Geometry: see drawing. Coordinates: mm, zero at the bounding-box minimum. Coordinates: 2 decimals unless noted, no trailing zeros. Order: outer loops, then holes, each group sorted by start corner. A loop starts at its lowest first (then second) coordinate and runs counter-clockwise, first axis right, second up. Notation, with made-up numbers: (-30.75, 47) -> (-16.75, 47) arc R17 ccw to (-16.75, 62) -> close; hole circle Ø2 at (33, -26.5). An arc over 180 degrees is marked (long way). Write each question's results on one line, items separated by ' | '.
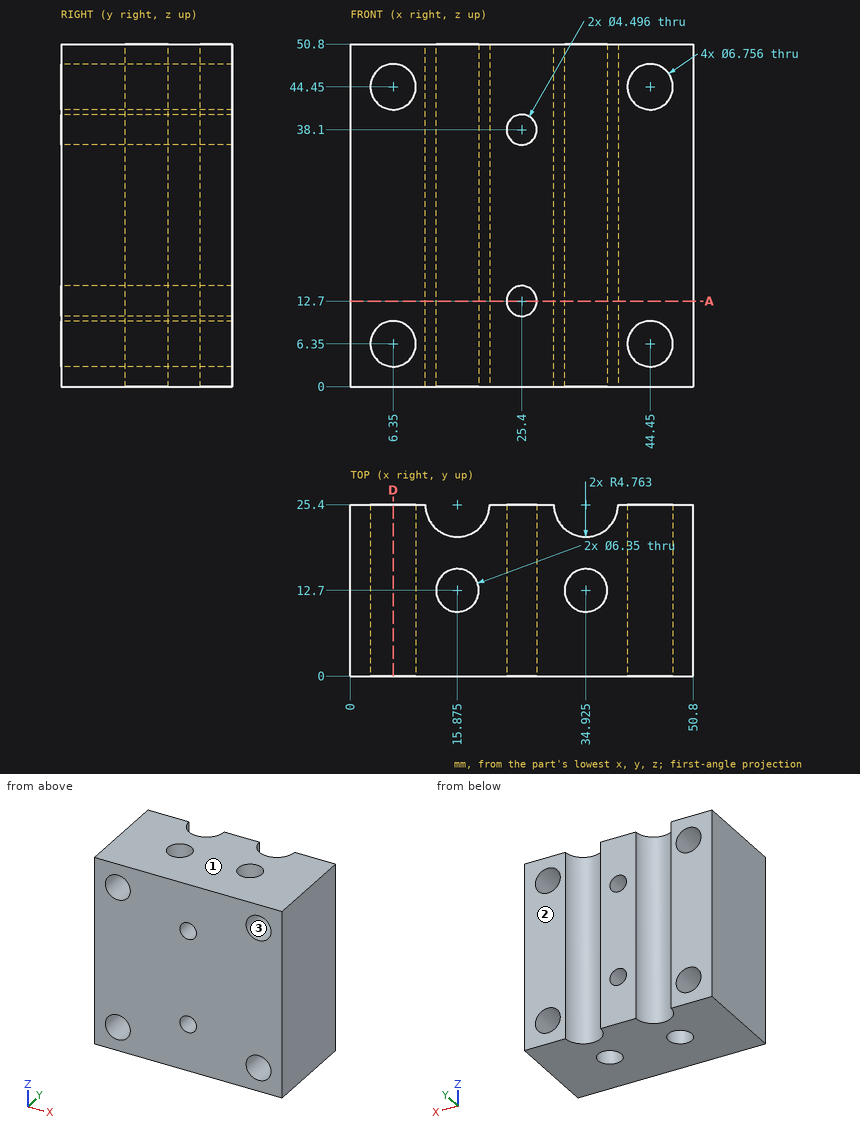
(1) Line query: line 1 along X through (y, z) = (19, 6.35); line 2 along Z through (x, y) = (25.4, 20.25). Output: solid intervals per line, ascending. Write a range as from..to.
Return value:
line 1: 0..2.97, 9.73..41.07, 47.83..50.8 | line 2: 0..10.45, 14.95..35.85, 40.35..50.8
(2) Cut plane D-D, the plane x = 6.35. Return loops of the section in (y, z), plus the area to 3 significant figures.
Return value:
outline: (0, 0) -> (25.4, 0) -> (25.4, 2.97) -> (0, 2.97) -> close; (0, 9.73) -> (25.4, 9.73) -> (25.4, 41.07) -> (0, 41.07) -> close; (0, 47.83) -> (25.4, 47.83) -> (25.4, 50.8) -> (0, 50.8) -> close | area: 947 mm2
(3) Cut plane A-A, the plane z = 12.7. Count the separate pieces of the cut face and the enclosed holes in it, plus the area to 3 significant figures.
Return value:
separate pieces: 2 | enclosed holes: 2 | area: 1,040 mm2
(4) Pin query (flat end, axial travel): P1, Ø12, axis at x = 40.5, y = 11.5, coming from the -Z side. Return the tip coordinate at first contact, or that it passes through.
Return value:
P1: z = 0
(5) Mould query, pull axis Z, two halves, no side actions, for the marked faces 1, 2 and 3. Classes: +Z half, -Z half, draft (parallel to the pull), parting line (faces both ways), or undercut.
Return value:
face 1: +Z half | face 2: draft | face 3: undercut
